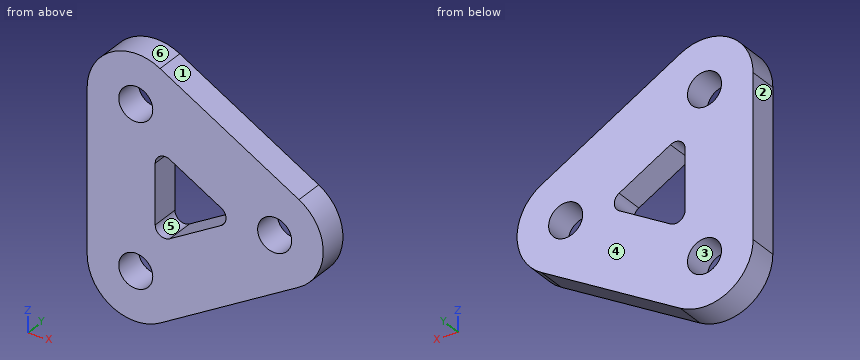
from build123d import *

# Parameters (mm, degrees)
SKETCH3_R           = 1.75
BOSS_EXTRUDE1_DEPTH = 3


with BuildPart() as part:
    # Sketch3 → Boss-Extrude1 (new body)
    with BuildSketch(Plane(origin=(0, 0, 0), x_dir=(1, 0, 0), z_dir=(0, 1, 0))):
        with BuildLine():
            Line((9.644709581, 4.330127019), (-4.644709581, 12.580127019))
            ThreePointArc((-4.644709581, 12.580127019), (-9.644709581, 12.580127019), (-12.144709581, 8.25))
            Line((-12.144709581, 8.25), (-12.144709581, -8.25))
            ThreePointArc((-12.144709581, -8.25), (-9.644709581, -12.580127019), (-4.644709581, -12.580127019))
            Line((-4.644709581, -12.580127019), (9.644709581, -4.330127019))
            ThreePointArc((9.644709581, -4.330127019), (12.144709581, 0), (9.644709581, 4.330127019))
        make_face()
        with Locations((7.144709581, 0)):
            Circle(SKETCH3_R, mode=Mode.SUBTRACT)
        with Locations((-7.144709581, 8.25)):
            Circle(SKETCH3_R, mode=Mode.SUBTRACT)
        with Locations((-7.144709581, -8.25)):
            Circle(SKETCH3_R, mode=Mode.SUBTRACT)
        with BuildLine():
            Line((1.644709581, 0.866025404), (-3.644709581, 3.919872981))
            ThreePointArc((-3.644709581, 3.919872981), (-4.644709581, 3.919872981), (-5.144709581, 3.053847577))
            Line((-5.144709581, 3.053847577), (-5.144709581, -3.053847577))
            ThreePointArc((-5.144709581, -3.053847577), (-4.644709581, -3.919872981), (-3.644709581, -3.919872981))
            Line((-3.644709581, -3.919872981), (1.644709581, -0.866025404))
            ThreePointArc((1.644709581, -0.866025404), (2.144709581, 0), (1.644709581, 0.866025404))
        make_face(mode=Mode.SUBTRACT)
    extrude(amount=BOSS_EXTRUDE1_DEPTH)


solid = part.part
CAD build for the part. Positions are in the model's coordinates, mm. Face numbers are marked on the shaded views. A direction names the side the tool comes from. Round coordinates to 2 decimals unless told otherwise and drop trailing zeros. Order: outer loops, then holes, each group sorted by start corner. A loop starts at its lowest first (then second) coordinate and runs counter-clockwise, first axis right, second up. Notation, with made-up numbers: (31, 37) -> (60, 37) arc R37 cw to (60, 74) -> close; hole circle Ø6 at (-21.75, 57.5). An arc over 180 degrees is marked (long way). Write item = value, one per line. Start each with the question number.
(1) Cut at D-D, the plane x = 7.25. List the corners of the cut face in (y, z).
(2) Cut at C-C, the plane z = 9.25. List the corners of the cut face in (x, y).
(3) Which spindle directions (+Z, -Z, +X, -X, +Y, -Y) get a long thin tool onto all of the face, cutting with end or side? Do the marked faces 5 and 6. Say none if no direction does.
(4) Probe line 1 (X direction, y = 2.35, z = 0); line 2 (X direction, y = 1.25, z = -8.25); line 3 (Z direction, x = -6.5, y = 1.9). List the from-to ranges inside material, lowest first. Write a range as [from, to].
(5) Cut at A-A, the plane z = 0. List the corners of the cut face in (x, y).
(6) Cut at B-B, the plane y = 2.1. List the corners of the cut face in (x, z).
(7) Pin check, flat tips, straight feed: P1, Ø4, axis at x = -7, z = 7, coming from the -Y side; P2, Ø1.5, axis at y = 1.5, z = 4, coming from the +X side. Stop position of each tip, or through.
(8) Pull direction X, two halves, no side cores. Call the marked faces 1, 2, 3 and 4: released by +X, released by -X, zero draft, split by the parting line, or undercut.
Model answer:
q1.outline = (0, -5.71) -> (3, -5.71) -> (3, -1.75) -> (0, -1.75) -> close; (0, 1.75) -> (3, 1.75) -> (3, 5.71) -> (0, 5.71) -> close
q2.outline = (-12.04, 0) -> (-8.58, 0) -> (-8.58, 3) -> (-12.04, 3) -> close; (-5.71, 0) -> (1.12, 0) -> (1.12, 3) -> (-5.71, 3) -> close
q3.face_5 = +Y, -Y
q3.face_6 = +Z, +Y, -Y
q4.line_1 = [-12.14, -5.14], [2.14, 5.39], [8.89, 12.14]
q4.line_2 = [-12.14, -8.89], [-5.39, 2.86]
q4.line_3 = [-13.21, -9.88], [-6.62, 6.62], [9.88, 13.21]
q5.outline = (-12.14, 0) -> (-5.14, 0) -> (-5.14, 3) -> (-12.14, 3) -> close; (2.14, 0) -> (5.39, 0) -> (5.39, 3) -> (2.14, 3) -> close; (8.89, 0) -> (12.14, 0) -> (12.14, 3) -> (8.89, 3) -> close
q6.outline = (-12.14, -8.25) arc R5 ccw to (-4.64, -12.58) -> (9.64, -4.33) arc R5 ccw to (9.64, 4.33) -> (-4.64, 12.58) arc R5 ccw to (-12.14, 8.25) -> close; hole circle Ø3.5 at (-7.14, -8.25); hole circle Ø3.5 at (-7.14, 8.25); hole (-5.14, -3.05) arc R1 ccw to (-3.64, -3.92) -> (1.64, -0.87) arc R1 ccw to (1.64, 0.87) -> (-3.64, 3.92) arc R1 ccw to (-5.14, 3.05) -> close; hole circle Ø3.5 at (7.14, 0)
q7.P1 = 0
q7.P2 = 10.94
q8.face_1 = released by +X
q8.face_2 = released by -X
q8.face_3 = undercut
q8.face_4 = zero draft
